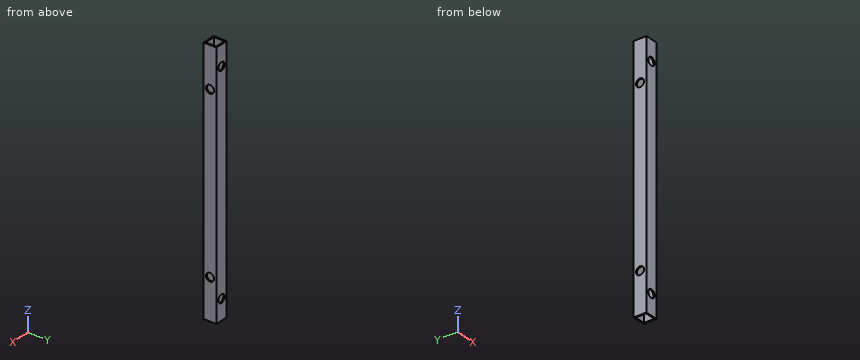
```python
from build123d import *

# Parameters (mm, degrees)
SKETCH_R         = 3.96875
EXTRUDE001_DEPTH = 12.7
SKETCH001_R      = 3.96875
EXTRUDE_DEPTH    = 12.7
BOX001_W         = 10.3
BOX001_H         = 10.3
BOX001_DEPTH     = 250
BOX_W            = 12.7
BOX_H            = 12.7
BOX_DEPTH        = 250


with BuildPart() as extrude001:
    # Sketch (on Face6 of Cut001) → Extrude001 (new body)
    with BuildSketch(Plane.YZ.offset(12.7)):
        with Locations((6.35, 210)):
            Circle(SKETCH_R)
        with Locations((6.35, 40)):
            Circle(SKETCH_R)
    extrude(amount=-EXTRUDE001_DEPTH)


with BuildPart() as extrude_body:
    # Sketch001 (on Face3 of Box) → Extrude (new body)
    with BuildSketch(Plane.XZ):
        with Locations((6.35, 20)):
            Circle(SKETCH001_R)
        with Locations((6.35, 230)):
            Circle(SKETCH001_R)
    extrude(amount=-EXTRUDE_DEPTH)


with BuildPart() as obj1:
    # Box001 → Box001 (new body)
    with BuildSketch(Plane(origin=(1.2, 1.2, 0), x_dir=(1, 0, 0), z_dir=(0, 0, 1))):
        with Locations((5.15, 5.15)):
            Rectangle(BOX001_W, BOX001_H)
    extrude(amount=BOX001_DEPTH)


with BuildPart() as cut002:
    # Box → Box (new body)
    with BuildSketch(Plane.XY):
        with Locations((6.35, 6.35)):
            Rectangle(BOX_W, BOX_H)
    extrude(amount=BOX_DEPTH)

    # Cut: cut obj1
    add(obj1.part, mode=Mode.SUBTRACT)

    # Cut001: cut Extrude body
    add(extrude_body.part, mode=Mode.SUBTRACT)

    # Cut002: cut Extrude001
    add(extrude001.part, mode=Mode.SUBTRACT)


solid = cut002.part
```
Read the model definition and answer for the solid it produces. Units are mm, in the model's axes. Give positions to 0.01 mm unless a question says otherwise; leave off trailing zeros. Loops run counter-clockwise (first coordinate to the right, second up) from the corner with the lowest first, then second, coordinate; pieces in that order, holes last.
Item 1: The part is cut by section B-B (y = 6.35). Write down the section's boundary in (x, z), and give its area (3 significant figures).
Item 2: The part is cut by section D-D (z = 143). Write down the section's boundary in (x, y), and give its area (3 significant figures).
Item 3: The part is cut by section A-A (z = 230). Write down the section's boundary in (x, y), and give its area (4 significant figures).
Item 4: Find the intervals of material crossed by line 1 along Z through (x, y) = (0.45, 6.35); line 2 along Z through (x, y) = (6.35, 0.75); line 3 along X through (y, z) = (3.5, 122.5), in increasing order.
Item 5: The part is cut by section C-C (x = 6.35). Write down the section's boundary in (y, z).
Item 6: This flat-tipped pin is pushed along its axis until it touches: pin 1 Ø5 at (y, z) = (6.35, 210) entering from +X. Where does it stop, or does it pass through?
Taken from the geometry:
1. outline: (0, 0) - (1.2, 0) - (1.2, 36.03) - (0, 36.03) - close; (0, 43.97) - (1.2, 43.97) - (1.2, 206.03) - (0, 206.03) - close; (0, 213.97) - (1.2, 213.97) - (1.2, 250) - (0, 250) - close; (11.5, 0) - (12.7, 0) - (12.7, 36.03) - (11.5, 36.03) - close; (11.5, 43.97) - (12.7, 43.97) - (12.7, 206.03) - (11.5, 206.03) - close; (11.5, 213.97) - (12.7, 213.97) - (12.7, 250) - (11.5, 250) - close
1. area: 562 mm2
2. outline: (0, 0) - (12.7, 0) - (12.7, 12.7) - (0, 12.7) - close; hole (1.2, 1.2) - (11.5, 1.2) - (11.5, 11.5) - (1.2, 11.5) - close
2. area: 55.2 mm2
3. outline: (0, 0) - (2.38, 0) - (2.38, 1.2) - (1.2, 1.2) - (1.2, 11.5) - (2.38, 11.5) - (2.38, 12.7) - (0, 12.7) - close; (10.32, 0) - (12.7, 0) - (12.7, 12.7) - (10.32, 12.7) - (10.32, 11.5) - (11.5, 11.5) - (11.5, 1.2) - (10.32, 1.2) - close
3. area: 36.15 mm2
4. line 1: z = 0 to 36.03, 43.97 to 206.03, 213.97 to 250
4. line 2: z = 0 to 16.03, 23.97 to 226.03, 233.97 to 250
4. line 3: x = 0 to 1.2, 11.5 to 12.7
5. outline: (0, 0) - (1.2, 0) - (1.2, 16.03) - (0, 16.03) - close; (0, 23.97) - (1.2, 23.97) - (1.2, 226.03) - (0, 226.03) - close; (0, 233.97) - (1.2, 233.97) - (1.2, 250) - (0, 250) - close; (11.5, 0) - (12.7, 0) - (12.7, 16.03) - (11.5, 16.03) - close; (11.5, 23.97) - (12.7, 23.97) - (12.7, 226.03) - (11.5, 226.03) - close; (11.5, 233.97) - (12.7, 233.97) - (12.7, 250) - (11.5, 250) - close
6. pin 1: passes through
